The listing builds one solid part. Answer for the finished solid, in the listing's coordinates (mm). Coordinates: 2 decimals unless noted, no trailing zeros. Write each loop counter-clockwise with the first axis right and the second up, starting at its lowest first coordinate (ties: lowest second). Pieces come first, ordered by that corner, then holes.
(1) The part is cut by section B-B on y = 9.25. Determine the outline of the cut face in (x, z).
(2) Given P1, Ø2.5, axis at x = 9, z = 5, coming from the +Y side; P2, Ø0.5, axis at y = 4, z = 6, coming from the +X side, each flat-ended and moving along its own axis, determine where each tip first touches the part or whether it passes through.
(3) The part is cut by section A-A on z = 5. Determine the outline of the cut face in (x, y) (3 decimals).
(4) The part is cut by section C-C on x = 13.5. Determine the outline of the cut face in (y, z).
(5) The part is cut by section D-D on z = 59. Determine the outline of the cut face in (x, y) (3 decimals).
(6) Straight lines are drawn through the part: line 1 (Z direction, x = 15.5, y = 4); line 2 (Z direction, x = 2.25, y = 4.75); line 3 (X direction, y = 1.8, z = 19.5). For each, find the intervals that lie inside material, in ascending order.
from build123d import *

# Parameters (mm, degrees)
SKETCH1_W           = 18
SKETCH1_H           = 10
BOSS_EXTRUDE2_DEPTH = 64
CUT_EXTRUDE1_REACH  = 69.231
SKETCH3_W           = 4.3
SKETCH3_H           = 3.7
SKETCH5_R           = 1.425
CUT_EXTRUDE3_DEPTH  = 4.5
SKETCH7_R           = 1.44113796
CUT_EXTRUDE5_DEPTH  = 10
SKETCH8_R           = 1.6
CUT_EXTRUDE6_DEPTH  = 10
SKETCH9_R           = 1.6
CUT_EXTRUDE7_DEPTH  = 42.5
SKETCH10_R          = 1.25
CUT_EXTRUDE8_DEPTH  = 6


with BuildPart() as part:
    # Sketch1 → Boss-Extrude2 (new body)
    with BuildSketch(Plane.XY):
        with Locations((9, 5)):
            Rectangle(SKETCH1_W, SKETCH1_H)
    extrude(amount=BOSS_EXTRUDE2_DEPTH)

    # Sketch3 → Cut-Extrude1 (cut, up to next)
    with BuildSketch(Plane(origin=(0, 0, 0), x_dir=(-1, 0, 0), z_dir=(0, 0, -1)), mode=Mode.PRIVATE) as cut_extrude1_sk1:
        with Locations((-9, 8.15)):
            Rectangle(SKETCH3_W, SKETCH3_H)
    cut_extrude1_tool1 = extrude(cut_extrude1_sk1.sketch, amount=-CUT_EXTRUDE1_REACH, mode=Mode.PRIVATE) & part.part
    add(cut_extrude1_tool1.solids().sort_by_distance((9, 8.15, 0))[0], mode=Mode.SUBTRACT)

    # Sketch5 → Cut-Extrude3 (cut)
    with BuildSketch(Plane(origin=(0, 6.3, 0), x_dir=(1, 0, 0), z_dir=(0, 1, 0))):
        with Locations(Location((9, -23, 0), (0, 0, 180))):
            Circle(SKETCH5_R)
        with Locations(Location((9, -41, 0), (0, 0, 180))):
            Circle(SKETCH5_R)
        with Locations(Location((9, -5, 0), (0, 0, 180))):
            Circle(SKETCH5_R)
        with Locations(Location((9, -59, 0), (0, 0, 180))):
            Circle(SKETCH5_R)
    extrude(amount=-CUT_EXTRUDE3_DEPTH, mode=Mode.SUBTRACT)

    # Sketch7 → Cut-Extrude5 (cut)
    with BuildSketch(Plane(origin=(18, 0, 0), x_dir=(0, 0, -1), z_dir=(1, 0, 0))):
        with Locations((-5, 4)):
            Circle(SKETCH7_R)
        with Locations((-59, 4)):
            Circle(SKETCH7_R)
    extrude(amount=-CUT_EXTRUDE5_DEPTH, mode=Mode.SUBTRACT)

    # Sketch8 → Cut-Extrude6 (cut)
    with BuildSketch(Plane.ZY):
        with Locations((23, 4)):
            Circle(SKETCH8_R)
        with Locations((41, 4)):
            Circle(SKETCH8_R)
    extrude(amount=-CUT_EXTRUDE6_DEPTH, mode=Mode.SUBTRACT)

    # Sketch9 → Cut-Extrude7 (cut)
    with BuildSketch(Plane(origin=(0, 0, 0), x_dir=(-1, 0, 0), z_dir=(0, 0, -1))):
        with Locations(Location((-4.5, 4, 0), (0, 0, 270))):
            Circle(SKETCH9_R)
    extrude(amount=-CUT_EXTRUDE7_DEPTH, mode=Mode.SUBTRACT)

    # Sketch10 → Cut-Extrude8 (cut)
    with BuildSketch(Plane.XZ):
        with Locations(Location((13.5, 19.5, 0), (0, 0, 270))):
            Circle(SKETCH10_R)
        with Locations(Location((13.5, 44.5, 0), (0, 0, 270))):
            Circle(SKETCH10_R)
    extrude(amount=-CUT_EXTRUDE8_DEPTH, mode=Mode.SUBTRACT)


solid = part.part
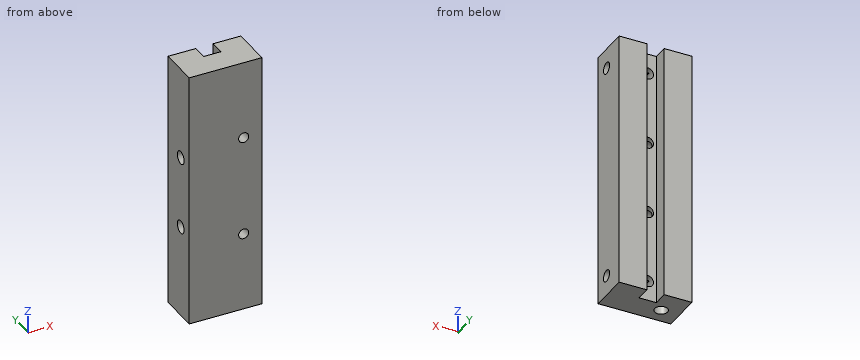
Model answer:
1. outline: (0, 0) - (6.85, 0) - (6.85, 64) - (0, 64) - close; (11.15, 0) - (18, 0) - (18, 64) - (11.15, 64) - close
2. P1: stops at y = 1.8
2. P2: stops at x = 8
3. outline: (0, 0) - (18, 0) - (18, 2.559) - (10.425, 2.559) - (10.425, 1.8) - (7.575, 1.8) - (7.575, 6.3) - (6.85, 6.3) - (6.85, 10) - (0, 10) - close; (10.425, 5.441) - (18, 5.441) - (18, 10) - (11.15, 10) - (11.15, 6.3) - (10.425, 6.3) - close; hole circle Ø3.2 at (4.5, 4)
4. outline: (0, 0) - (10, 0) - (10, 64) - (0, 64) - (0, 45.75) - (6, 45.75) - (6, 43.25) - (0, 43.25) - (0, 20.75) - (6, 20.75) - (6, 18.25) - (0, 18.25) - close; hole circle Ø2.88 at (4, 5); hole circle Ø2.88 at (4, 59)
5. outline: (0, 0) - (18, 0) - (18, 2.559) - (10.425, 2.559) - (10.425, 1.8) - (7.575, 1.8) - (7.575, 6.3) - (6.85, 6.3) - (6.85, 10) - (0, 10) - close; (10.425, 5.441) - (18, 5.441) - (18, 10) - (11.15, 10) - (11.15, 6.3) - (10.425, 6.3) - close
6. line 1: z = 0 to 3.56, 6.44 to 57.56, 60.44 to 64
6. line 2: z = 0 to 21.59, 24.41 to 39.59, 42.41 to 64
6. line 3: x = 0 to 12.25, 14.75 to 18
